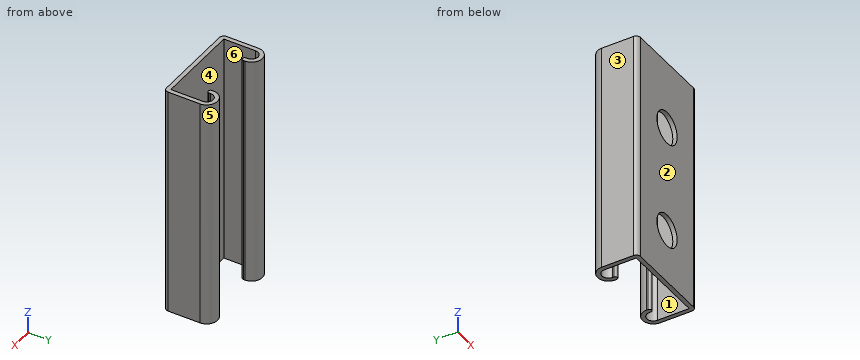
from build123d import *

# Parameters (mm, degrees)
BASE_EXTRUDE_DEPTH = 101.6
HOLE1_START        = -8.4582
HOLE1_OUTLINE_R    = 7.14375
HOLE1_DEPTH        = 1.905
LPATTERN2_COUNT    = 2
LPATTERN2_PITCH    = 47.625


with BuildPart() as part:
    # Sketch1 → Base-Extrude (new body)
    with BuildSketch(Plane.XY):
        with BuildLine():
            Line((-20.6375, 7.4295), (-20.6375, -6.5532))
            ThreePointArc((-20.6375, -6.5532), (-20.079538418, -7.900238418), (-18.7325, -8.4582))
            Line((-18.7325, -8.4582), (18.7325, -8.4582))
            ThreePointArc((18.7325, -8.4582), (20.079538418, -7.900238418), (20.6375, -6.5532))
            Line((20.6375, -6.5532), (20.6375, 7.4295))
            ThreePointArc((20.6375, 7.4295), (15.875, 12.192), (11.1125, 7.4295))
            Line((11.1125, 7.4295), (11.1125, 6.7945))
            ThreePointArc((11.1125, 6.7945), (12.065, 5.842), (13.0175, 6.7945))
            Line((13.0175, 6.7945), (13.0175, 7.4295))
            ThreePointArc((13.0175, 7.4295), (15.875, 10.287), (18.7325, 7.4295))
            Line((18.7325, 7.4295), (18.7325, -6.5532))
            Line((18.7325, -6.5532), (-18.7325, -6.5532))
            Line((-18.7325, -6.5532), (-18.7325, 7.4295))
            ThreePointArc((-18.7325, 7.4295), (-15.875, 10.287), (-13.0175, 7.4295))
            Line((-13.0175, 7.4295), (-13.0175, 6.7945))
            ThreePointArc((-13.0175, 6.7945), (-12.065, 5.842), (-11.1125, 6.7945))
            Line((-11.1125, 6.7945), (-11.1125, 7.4295))
            ThreePointArc((-11.1125, 7.4295), (-15.875, 12.192), (-20.6375, 7.4295))
        make_face()
    extrude(amount=BASE_EXTRUDE_DEPTH)

    # Hole1: read off the stored shape, not the designer's step
    # Hole1 outline → Hole1 (cut)
    with BuildSketch(Plane(origin=(0, 0, 0), x_dir=(1, 0, 0), z_dir=(0, 1, 0)).offset(HOLE1_START)):
        with Locations((0, -23.8125)):
            Circle(HOLE1_OUTLINE_R)
    hole1 = extrude(amount=HOLE1_DEPTH, mode=Mode.SUBTRACT)

    # LPattern2: Hole1 ×2
    with Locations(*[(0, 0, i * LPATTERN2_PITCH) for i in range(1, LPATTERN2_COUNT)]):
        add(hole1, mode=Mode.SUBTRACT)


solid = part.part
Source: CAD feature listing. Evaluate the final solid. Frame: model axes, mm. Face numbers are marked on the shaded views. A direction names the side the tool comes from. Give positions to 0.01 mm unless a question says otherwise; leave off trailing zeros. Write each loop counter-clockwise with the first axis right and the second up, starting at its lowest first coordinate (ties: lowest second). Pieces come first, ordered by that corner, then holes. Notation, with made-up numbers: M -25.75,-17.75 L -6.75,-17.75 A18 ccw -6.75,-7.75 Z; hole C 30,27 d6. An arc over 180 degrees is marked long. Answer as a JSON object with one key per item and string values.
Q1. Mould query, pull axis X, two halves, no side actions, for the marked faces 1, 2, 3 and 4. Classes: +X half, -X half, draft (parallel to the pull), parting line (faces both ways), or undercut.
Geometry check:
{"face 1": "undercut", "face 2": "draft", "face 3": "-X half", "face 4": "undercut"}
Q2. Cut plane A-A, the plane x = 0. Return the cut outline in (y, z).
Geometry check:
{"outline": "M -8.46,0 L -6.55,0 L -6.55,16.67 L -8.46,16.67 Z; M -8.46,30.96 L -6.55,30.96 L -6.55,64.29 L -8.46,64.29 Z; M -8.46,78.58 L -6.55,78.58 L -6.55,101.6 L -8.46,101.6 Z"}
Q3. Ray query, line 1 along Z through (x, y) = (0, -7.2); line 2 along X through (y, z) = (1.5, 8); line 3 along Y through (x, z) = (-16, 53). Return the intervals inside material, ascending.
Geometry check:
{"line 1": "z = 0 to 16.67, 30.96 to 64.29, 78.58 to 101.6", "line 2": "x = -20.64 to -18.73, 18.73 to 20.64", "line 3": "y = -8.46 to -6.55, 10.28 to 12.19"}
Q4. Cut plane C-C, the plane z = 76. Return the cut outline in (x, y) (1 decimal).
Geometry check:
{"outline": "M -20.6,-6.6 A1.9 ccw -18.7,-8.5 L -5.5,-8.5 L -5.5,-6.6 L -18.7,-6.6 L -18.7,7.4 A2.9 cw -13,7.4 L -13,6.8 A1 ccw -11.1,6.8 L -11.1,7.4 A4.8 ccw -20.6,7.4 Z; M 5.5,-8.5 L 18.7,-8.5 A1.9 ccw 20.6,-6.6 L 20.6,7.4 A4.8 ccw 11.1,7.4 L 11.1,6.8 A1 ccw 13,6.8 L 13,7.4 A2.9 cw 18.7,7.4 L 18.7,-6.6 L 5.5,-6.6 Z"}
Q5. Access query for the marked faces 5 and 6. Directions: +Z, -Z, +X, -X, +Y, -Y. A direction counts if a zero-diameter tool reaches every point of the face in a straight line with its end or side. Return the directions, or none.
Geometry check:
{"face 5": "+Z, -Z, +Y", "face 6": "+Z, -Z"}
Q6. Cut plane D-D, the plane z = 35. Return the cut outline in (x, y) (1 decimal), then the cut area to 3 significant figures.
Geometry check:
{"outline": "M -20.6,-6.6 A1.9 ccw -18.7,-8.5 L 18.7,-8.5 A1.9 ccw 20.6,-6.6 L 20.6,7.4 A4.8 ccw 11.1,7.4 L 11.1,6.8 A1 ccw 13,6.8 L 13,7.4 A2.9 cw 18.7,7.4 L 18.7,-6.6 L -18.7,-6.6 L -18.7,7.4 A2.9 cw -13,7.4 L -13,6.8 A1 ccw -11.1,6.8 L -11.1,7.4 A4.8 ccw -20.6,7.4 Z", "area": "181 mm^2"}
Q7. Contact query for flat-ended pins moving along their axis: P1, Ø23, axis at x = 0, z = 23.81, coming from the -Y side; P2, Ø11, axis at x = 3.5, z = 53.5, coming from the +Y side; P3, Ø2, axis at y = 10, z = 33, coming from the +X side; P4, Ø23, axis at x = 0, z = 71.44, coming from the +Y side. Output: stop coordinate, or through.
Geometry check:
{"P1": "stops at y = -8.46", "P2": "stops at y = -6.55", "P3": "stops at x = 20.37", "P4": "stops at y = 9.31"}
Q8. Cut plane B-B, the plane y = -4.5. Return the cut outline in (x, z).
Geometry check:
{"outline": "M -20.64,0 L -18.73,0 L -18.73,101.6 L -20.64,101.6 Z; M 18.73,0 L 20.64,0 L 20.64,101.6 L 18.73,101.6 Z"}
